The model under review builds one solid part; all positions refer to its coordinate system, in mm. A direction names the side the tool comes from. Coordinates: 2 decimals unless noted, no trailing zeros. Write each loop counter-clockwise with the first axis right and the second up, starting at its lowest first coordinate (ties: lowest second). Pieces come first, ordered by that corner, then holes.
```python
from build123d import *

# Parameters (mm, degrees)
F0_W     = 138.7
F0_H     = 47
F1_DEPTH = 26
F2_W     = 8.5
F2_H     = 47
F2_R     = 2.5
F2_R_2   = 0.93
F3_DEPTH = 2
F2_R_3   = 0.8
F2_R_4   = 2
F4_DEPTH = 15


with BuildPart() as f1:
    # F0 (on Front) → F1 (new body)
    with BuildSketch(Plane.XZ):
        Rectangle(F0_W, F0_H)
    extrude(amount=F1_DEPTH)

    # F2 (on face) → F3 (cut)
    with BuildSketch(Plane.XZ.offset(26)):
        with Locations((65.1, 0)):
            Rectangle(F2_W, F2_H)
        with Locations((66.75, -17.5)):
            Circle(F2_R, mode=Mode.SUBTRACT)
        with Locations((66.85, 0)):
            Circle(F2_R_2, mode=Mode.SUBTRACT)
        with Locations((66.75, 17.5)):
            Circle(F2_R, mode=Mode.SUBTRACT)
    extrude(amount=-F3_DEPTH, mode=Mode.SUBTRACT)

    # F2 (on face) → F4 (cut)
    with BuildSketch(Plane.XZ.offset(26)):
        with Locations((66.85, 0)):
            Circle(F2_R_3)
        with Locations((66.75, 17.5)):
            Circle(F2_R_4)
        with Locations((66.75, -17.5)):
            Circle(F2_R_4)
    extrude(amount=-F4_DEPTH, mode=Mode.SUBTRACT)


solid = f1.part
```
Item 1: To check wall thickness, follow line 1 along Z through (x, y) = (66.75, -14.75). State the ranges of the line that lie inside material, in increasing order.
Solved:
line 1: z = -23.5 to -19.5, -15.5 to -0.79, 0.79 to 15.5, 19.5 to 23.5
Item 2: Mouldability with a two-part tool opening along X and no side actions: class faces 1 (the face through (69.135, -25.014, -16.749)), 2 (the face through (69.35, -12, 0)), 3 (the face through (-1, 0, 0)) as pulls with the +X half, pulls with the -X half, needs draft (parallel to the pull), parting line crosses it, or undercut.
Solved:
face 1: undercut
face 2: pulls with the +X half
face 3: needs draft
Item 3: For pin 1 (1.3 mm diameter, centred on x = 66.85, z = 0, fed in from -Y); pin 2 (4 mm diameter, centred on x = 64.5, z = -4.5, fed in from -Y); pin 3 (1.6 mm diameter, centred on y = -25.5, z = -6.5, fed in from +X), all flat-tipped, find the tip position at first contact; note any pin that passes through.
Solved:
pin 1: stops at y = -11
pin 2: stops at y = -24
pin 3: stops at x = 60.85
Item 4: Take a section at A-A, the plane z = -17.5. Write out the cut boundary in (x, y), plus the area to 3 significant figures.
Solved:
outline: (-69.35, -26) - (60.85, -26) - (60.85, -24) - (64.25, -24) - (64.25, -26) - (64.75, -26) - (64.75, -11) - (68.75, -11) - (68.75, -26) - (69.25, -26) - (69.25, -24) - (69.35, -24) - (69.35, 0) - (-69.35, 0) - close
area: 3,540 mm2
Item 5: Machinability: for faces 4 (the face through (-5, -26, 0)), 5 (the face through (67, -11, -17)), which of the approach directions +Z, -Z, +X, -X, +Y, -Y give a long, thin tool a straight path to every point of the face, cutting with its end or side? Answer none if there is none.
Solved:
face 4: +Z, -Z, +X, -X, -Y
face 5: -Y
